Model file for the job. Use its own axes, mm. A direction names the side the tool comes from. Give positions to 0.01 mm unless a question says otherwise; leave off trailing zeros. Write each loop counter-clockwise with the first axis right and the second up, starting at its lowest first coordinate (ties: lowest second). Pieces come first, ordered by that corner, then holes.
```python
from build123d import *

# Parameters (mm, degrees)
F0_W      = 73.406
F0_H      = 31.75
F1_DEPTH  = 14.224
F2_W      = 15.748
F2_H      = 28.575
F3_DEPTH  = 104.648
F5_DEPTH  = 22.099
F7_DEPTH  = 12.7
F8_W      = 6.35
F8_H      = 28.575
F9_DEPTH  = 4.826
F11_DEPTH = 22.099


with BuildPart() as f1:
    # F0 (on Front) → F1 (new body, symmetric)
    with BuildSketch(Plane.XZ):
        Rectangle(F0_W, F0_H)
    extrude(amount=F1_DEPTH, both=True)

    # F2 (on face) → F3 (join)
    with BuildSketch(Plane(origin=(-36.703, 0, 0), x_dir=(0, -1, 0), z_dir=(-1, 0, 0))):
        with Locations((0, 30.1625)):
            Rectangle(F2_W, F2_H)
    extrude(amount=-F3_DEPTH)

    # F4 (on face) → F5 (cut, through all)
    with BuildSketch(Plane.XZ.offset(7.874)):
        Polygon((67.945, 15.875), (67.945, 44.45), (39.37, 15.875), align=None)
    extrude(amount=-F5_DEPTH, mode=Mode.SUBTRACT)

    # F6 (on Front) → F7 (join, symmetric)
    with BuildSketch(Plane.XZ):
        Polygon((50.419, 26.924), (67.945, 44.45), (32.893, 44.45), (32.893, 26.924), align=None)
    extrude(amount=F7_DEPTH, both=True)

    # F8 (on face) → F9 (cut)
    with BuildSketch(Plane.XZ.offset(7.874)):
        with Locations((-33.528, 30.1625)):
            Rectangle(F8_W, F8_H)
    extrude(amount=-F9_DEPTH, mode=Mode.SUBTRACT)

    # F10 (on face) → F11 (cut, through all)
    with BuildSketch(Plane.XZ.offset(7.874)):
        with BuildLine():
            Line((-11.938, 24.511), (11.938, 24.511))
            ThreePointArc((11.938, 24.511), (6.35, 30.099), (11.938, 35.687))
            Line((11.938, 35.687), (-11.938, 35.687))
            ThreePointArc((-11.938, 35.687), (-7.986687, 34.050313), (-6.35, 30.099))
            ThreePointArc((-6.35, 30.099), (-7.986687, 26.147687), (-11.938, 24.511))
        make_face()
        with BuildLine():
            ThreePointArc((11.938, 35.687), (6.35, 30.099), (11.938, 24.511))
            ThreePointArc((11.938, 24.511), (15.889313, 26.147687), (17.526, 30.099))
            ThreePointArc((17.526, 30.099), (15.889313, 34.050313), (11.938, 35.687))
        make_face()
        with BuildLine():
            ThreePointArc((-11.938, 35.687), (-17.526, 30.099), (-11.938, 24.511))
            ThreePointArc((-11.938, 24.511), (-7.986687, 26.147687), (-6.35, 30.099))
            ThreePointArc((-6.35, 30.099), (-7.986687, 34.050313), (-11.938, 35.687))
        make_face()
    extrude(amount=-F11_DEPTH, mode=Mode.SUBTRACT)

    # F12: F1 across plane


with BuildPart() as f1_1:
    add(f1.part)
    add(f1.part.mirror(Plane.XY))


solid = f1_1.part
```
1. Probe probe 1 along Z at (x, y) = (-10, -6.25); probe 2 along Y at (x, z) = (2, -18); probe 3 along Z at (x, y) = (29, -12.25) (3 decimals). List the from-to ranges inside material, lowest first.
Calculated:
probe 1: z = -44.45 to -35.69, -24.51 to 24.51, 35.69 to 44.45
probe 2: y = -7.87 to 7.87
probe 3: z = -15.875 to 15.875
2. Pin check, flat tips, straight feed: P1, Ø2.5, axis at y = -9.5, z = 32, coming from the -X side; P2, Ø9, axis at x = 56, z = 37.5, coming from the +Y side; P3, Ø3, axis at x = 39, z = -4.5, coming from the +Y side; P4, Ø5.5, axis at y = 10.5, z = 38.5, coming from the -X side. Stop position of each tip, or through.
Calculated:
P1: stops at x = 32.89
P2: stops at y = 12.7
P3: passes through
P4: stops at x = -36.7
3. Slice it at A-A, the plane x = 38. Write the cut outline in (y, z) (3 decimals).
Calculated:
outline: (-12.7, -44.45) - (12.7, -44.45) - (12.7, -26.924) - (7.874, -26.924) - (7.874, -15.875) - (-7.874, -15.875) - (-7.874, -26.924) - (-12.7, -26.924) - close; (-12.7, 26.924) - (-7.874, 26.924) - (-7.874, 15.875) - (7.874, 15.875) - (7.874, 26.924) - (12.7, 26.924) - (12.7, 44.45) - (-12.7, 44.45) - close
4. Which spindle directions (+Z, -Z, +X, -X, +Y, -Y) get a long thin tool onto all of the face, cutting with end or side? Do faces 5 (the flat face through (46, 12.7, 36)), 6 (the flat face through (32.893, -10, -36)), 7 (the flat face through (32.893, 10, 36)). Say none if no direction does.
Calculated:
face 5: +Z, +X, -X, +Y
face 6: -Z, -X, -Y
face 7: +Z, -X, +Y
5. Slice it at D-D, the plane x = 24.5. Write the cut outline in (y, z) (3 decimals).
Calculated:
outline: (-14.224, -15.875) - (-7.874, -15.875) - (-7.874, -44.45) - (7.874, -44.45) - (7.874, -15.875) - (14.224, -15.875) - (14.224, 15.875) - (7.874, 15.875) - (7.874, 44.45) - (-7.874, 44.45) - (-7.874, 15.875) - (-14.224, 15.875) - close
6. Pull direction Z, two halves, no side cores. Call faces 1 (the flat face through (28, 0, 44.45)), 2 (the flat face through (56.632, -0.178, -33.137)), 3 (the flat face through (42, -10, 26.924)), 4 (the flat face through (-1, -14.224, 0)): +Z half, -Z half, draft (parallel to the pull), parting line (faces both ways), or undercut.
Calculated:
face 1: +Z half
face 2: undercut
face 3: undercut
face 4: draft
7. Slice it at B-B, the plane y = -6. Write the cut outline in (x, z) (3 decimals), and give its area (3 significant figures).
Calculated:
outline: (-36.703, -15.875) - (-30.353, -15.875) - (-30.353, -44.45) - (67.945, -44.45) - (39.37, -15.875) - (36.703, -15.875) - (36.703, 15.875) - (39.37, 15.875) - (67.945, 44.45) - (-30.353, 44.45) - (-30.353, 15.875) - (-36.703, 15.875) - close; hole (-11.938, -35.687) - (11.938, -35.687) arc R5.588 ccw to (17.526, -30.099) arc R5.588 ccw to (11.938, -24.511) - (-11.938, -24.511) arc R5.588 ccw to start; hole (-11.938, 24.511) - (11.938, 24.511) arc R5.588 ccw to (17.526, 30.099) arc R5.588 ccw to (11.938, 35.687) - (-11.938, 35.687) arc R5.588 ccw to start
area: 6,400 mm2
8. Slice it at C-C, the plane y = -11.5. Write the cut outline in (x, z) (3 decimals).
Calculated:
outline: (-36.703, -15.875) - (36.703, -15.875) - (36.703, 15.875) - (-36.703, 15.875) - close; (32.893, -44.45) - (67.945, -44.45) - (50.419, -26.924) - (32.893, -26.924) - close; (32.893, 26.924) - (50.419, 26.924) - (67.945, 44.45) - (32.893, 44.45) - close
